```python
from build123d import *

# Parameters (mm, degrees)
BOX003_W     = 10
BOX003_H     = 5.1
BOX003_DEPTH = 25
BOX002_W     = 10
BOX002_H     = 5.1
BOX002_DEPTH = 25
BOX001_W     = 10
BOX001_H     = 120
BOX001_DEPTH = 35
BOX_W        = 10
BOX_H        = 99
BOX_DEPTH    = 140


with BuildPart() as cube003:
    # Box003 → Box003 (new body)
    with BuildSketch(Plane(origin=(0, 99, 75), x_dir=(1, 0, 0), z_dir=(0, 0, 1))):
        with Locations((5, 2.55)):
            Rectangle(BOX003_W, BOX003_H)
    extrude(amount=BOX003_DEPTH)


with BuildPart() as cube002:
    # Box002 → Box002 (new body)
    with BuildSketch(Plane(origin=(0, -5.1, 75), x_dir=(1, 0, 0), z_dir=(0, 0, 1))):
        with Locations((5, 2.55)):
            Rectangle(BOX002_W, BOX002_H)
    extrude(amount=BOX002_DEPTH)


with BuildPart() as cut001:
    # Box001 → Box001 (new body)
    with BuildSketch(Plane(origin=(0, -10, 75), x_dir=(1, 0, 0), z_dir=(0, 0, 1))):
        with Locations((5, 60)):
            Rectangle(BOX001_W, BOX001_H)
    extrude(amount=BOX001_DEPTH)

    # Cut: cut Cube002
    add(cube002.part, mode=Mode.SUBTRACT)

    # Cut001: cut Cube003
    add(cube003.part, mode=Mode.SUBTRACT)


with BuildPart() as fusion:
    # Box → Box (new body)
    with BuildSketch(Plane.XY.offset(-30)):
        with Locations((5, 49.5)):
            Rectangle(BOX_W, BOX_H)
    extrude(amount=BOX_DEPTH)

    # Fusion: union Cut001
    add(cut001.part)


solid = fusion.part
```
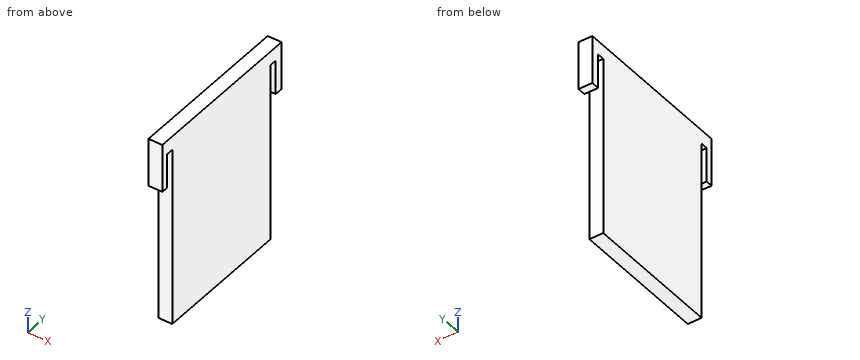
Build history of the part. All positions in model axes, mm. Coordinates: 2 decimals unless noted, no trailing zeros. Order: outer loops, then holes, each group sorted by start corner. A loop starts at its lowest first (then second) coordinate and runs counter-clockwise, first axis right, second up. Notation, with made-up numbers: (39, -14) -> (57, -14) arc R18 ccw to (57, 0) -> close; hole circle Ø8 at (49, 10.5). An arc over 180 degrees is marked (long way). Answer in a Markdown table with one row per item. Add a question column.
Q1. Drop flat-ended pins along their axis: pin 1 (3 mm diameter, centred on x = 4, z = 11, fed in from +Y); pin 2 (5 mm diameter, centred on x = 8.5, z = 71.5, fed in from -Y); pin 3 (5.5 mm diameter, centred on x = 3.5, y = -6.5, fed in from -Z). Give the stop position or say it passes through.
Q2. Band-saw the part on A-A, the plane z = 89.5. List the corners of the cut face in (x, y), then the cut area to 3 significant figures.
Q3. Wall check: line 1 along Y through (x, z) = (4.25, 95.5); line 2 along Y through (x, z) = (8, 23.5); line 3 along Z through (x, y) = (9.5, 104.5). Give the ranges that are in metal, low to high. Write a range as [from, to].
Q4. Band-saw the part on C-C, the plane z = 16. List the corners of the cut face in (x, y).
Q5. Band-saw the part on B-B, the plane x = 4.25. List the corners of the cut face in (y, z).
Answers follow:
| question | item | result |
|---|---|---|
| 1 | pin 1 | y = 99 |
| 1 | pin 2 | y = 0 |
| 1 | pin 3 | z = 75 |
| 2 | outline | (0, -10) -> (10, -10) -> (10, -5.1) -> (0, -5.1) -> close; (0, 0) -> (10, 0) -> (10, 99) -> (0, 99) -> close; (0, 104.1) -> (10, 104.1) -> (10, 110) -> (0, 110) -> close |
| 2 | area | 1,100 mm^2 |
| 3 | line 1 | [-10, -5.1], [0, 99], [104.1, 110] |
| 3 | line 2 | [0, 99] |
| 3 | line 3 | [75, 110] |
| 4 | outline | (0, 0) -> (10, 0) -> (10, 99) -> (0, 99) -> close |
| 5 | outline | (-10, 75) -> (-5.1, 75) -> (-5.1, 100) -> (0, 100) -> (0, -30) -> (99, -30) -> (99, 100) -> (104.1, 100) -> (104.1, 75) -> (110, 75) -> (110, 110) -> (-10, 110) -> close |
